```python
from build123d import *

# Parameters (mm, degrees)
SKETCH1_W           = 1900
SKETCH1_H           = 950
BOSS_EXTRUDE1_DEPTH = 30
BOSS_EXTRUDE2_DEPTH = 350
BOSS_EXTRUDE4_DEPTH = 30
SKETCH3_W           = 400
SKETCH3_H           = 100
BOSS_EXTRUDE5_DEPTH = 10


with BuildPart() as part:
    # Sketch1 → Boss-Extrude1 (new body)
    with BuildSketch(Plane(origin=(0, 0, 0), x_dir=(1, 0, 0), z_dir=(0, 1, 0))):
        with Locations((950, -475)):
            Rectangle(SKETCH1_W, SKETCH1_H)
    extrude(amount=BOSS_EXTRUDE1_DEPTH)

    # Sketch1_3 → Boss-Extrude2 (add)
    with BuildSketch(Plane(origin=(0, 0, 0), x_dir=(1, 0, 0), z_dir=(0, 1, 0))):
        Polygon((0, 0), (0, -10), (1890, -10), (1890, -950), (1900, -950), (1900, 0), align=None)
    extrude(amount=BOSS_EXTRUDE2_DEPTH)

    # Sketch1_4 → Boss-Extrude4 (add)
    with BuildSketch(Plane(origin=(0, 0, 0), x_dir=(1, 0, 0), z_dir=(0, 1, 0))):
        Polygon((1900, -950), (1890, -950), (400, -950), (400, -1450), (1900, -1450), align=None)
    extrude(amount=BOSS_EXTRUDE4_DEPTH)

    # Sketch3 → Boss-Extrude5 (add)
    with BuildSketch(Plane.XY.offset(950)):
        with BuildLine():
            ThreePointArc((400, 130), (464.436508139, 285.563491861), (620, 350))
            Line((620, 350), (1900, 350))
            Line((1900, 350), (1900, 30))
            Line((1900, 30), (400, 30))
            Line((400, 30), (400, 130))
        make_face()
        with Locations((200, 80)):
            Rectangle(SKETCH3_W, SKETCH3_H)
    extrude(amount=-BOSS_EXTRUDE5_DEPTH)


solid = part.part
```
The listing builds one solid part. Answer for the finished solid, in the listing's coordinates (mm). A direction names the side the tool comes from. Round coordinates to 2 decimals unless told otherwise and drop trailing zeros. Write each loop counter-clockwise with the first axis right and the second up, starting at its lowest first coordinate (ties: lowest second). Pieces come first, ordered by that corner, then holes. Notation, with made-up numbers: (56.5, 66) -> (109.5, 66) arc R16 cw to (109.5, 96) -> close; hole circle Ø5 at (-13.75, 63.25). An arc over 180 degrees is marked (long way). Use CSV: the item, a comma, the result in double quotes. Start each with the question number.
(1) Which of the six approach directions +Z, -Z, +X, -X, +Y, -Y give full straight-line access (tool end or side, diameter ignored) to faces 4 (the face through (932, 30, 468)), 5 (the face through (1140, 30, 1196)), 6 (the face through (462.735, 283.844, 945.07))?
(2) Section D-D on x = 251 is taken. Give the vertices of the cut face in (y, z).
(3) Section C-C on y = 237.5 is taken. Give the vertices of the cut face in (x, z), then the cut area to 3 significant figures.
(4) The mould has two halves that part along Z. Classify faces 1 (the face through (1168, 192, 940)), 2 (the face through (937, 173, 0)), 3 (the face through (1900, 173, 574)): released by +Z, released by -Z, zero draft, split by the parting line, or undercut.
(5) Consider L1, parallel to Z at x = 616.5, y = 246; L2, parallel to X at y = 156.5, z = 708.5; L3, parallel to Y at x = 1017.5, z = 543.5. Determine where each line is inside the solid, lowest interval first. Write a range as from..to.
(6) Section A-A on x = 1031.5 is taken. Give the vertices of the cut face in (y, z), then the cut area to 3 significant figures.
(7) Each of these flat-tipped pins is pushed along its axis until it touches: pin 1 (12 mm diameter, centred on x = 618, y = 250, fed in from +Z); pin 2 (2 mm diameter, centred on x = 572, y = 283.5, fed in from -Z); pin 3 (12 mm diameter, centred on x = 1266.5, z = 509, fed in from +Y); pin 4 (8 mm diameter, centred on x = 210, z = 943.5, fed in from +Y). Where does it stop, or does it pass through?
(8) Section B-B on z = 246 is taken. Give the vertices of the cut face in (x, y).
A:
1,face 4,"-X, +Y"
1,face 5,"+Z, +X, -X, +Y"
1,face 6,"+Z, -X, +Y"
2,outline,"(0, 0) -> (350, 0) -> (350, 10) -> (30, 10) -> (30, 940) -> (130, 940) -> (130, 950) -> (0, 950) -> close"
3,outline,"(0, 0) -> (1900, 0) -> (1900, 950) -> (428.05, 950) -> (428.05, 940) -> (1890, 940) -> (1890, 10) -> (0, 10) -> close"
3,area,"43,000 mm²"
4,face 1,"undercut"
4,face 2,"released by -Z"
4,face 3,"zero draft"
5,L1,"z = 0..10, 940..950"
5,L2,"x = 1890..1900"
5,L3,"y = 0..30"
6,outline,"(0, 0) -> (350, 0) -> (350, 10) -> (30, 10) -> (30, 940) -> (350, 940) -> (350, 950) -> (30, 950) -> (30, 1450) -> (0, 1450) -> close"
6,area,"49,900 mm²"
7,pin 1,"stops at z = 950"
7,pin 2,"stops at z = 0"
7,pin 3,"stops at y = 30"
7,pin 4,"stops at y = 130"
8,outline,"(0, 0) -> (1900, 0) -> (1900, 350) -> (1890, 350) -> (1890, 30) -> (0, 30) -> close"
